Check sheet for the modelled part. Datum: model origin and axes. Units: mm. Round coordinates to 2 decimals unless told otherwise and drop trailing zeros. Loops run counter-clockwise (first coordinate to the right, second up) from the corner with the lowest first, then second, coordinate; pieces in that order, holes last. Notation, with made-up numbers: (67, -7) -> (106, -7) arc R21 ccw to (106, 29) -> close; hole circle Ø11 at (24, 15.5). An arc over 180 degrees is marked (long way). Return JSON: item names as keys, results as strings.
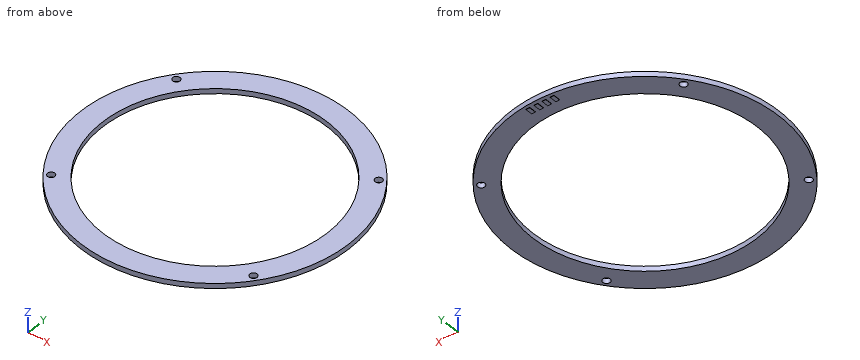
from build123d import *

# Parameters (mm, degrees)
SKETCH1_R           = 43
SKETCH1_R_2         = 36
SKETCH1_R_3         = 1.15
BOSS_EXTRUDE2_DEPTH = 1.6
SKETCH4_W           = 1.2
SKETCH4_H           = 2.3
BOSS_EXTRUDE3_DEPTH = 0.1


with BuildPart() as part:
    # Sketch1 → Boss-Extrude2 (new body)
    with BuildSketch(Plane.XY):
        Circle(SKETCH1_R)
        Circle(SKETCH1_R_2, mode=Mode.SUBTRACT)
        with Locations((32.5, -24.9)):
            Circle(SKETCH1_R_3, mode=Mode.SUBTRACT)
        with Locations((-32.5, -24.9)):
            Circle(SKETCH1_R_3, mode=Mode.SUBTRACT)
        with Locations((-32.5, 24.9)):
            Circle(SKETCH1_R_3, mode=Mode.SUBTRACT)
        with Locations((32.5, 24.9)):
            Circle(SKETCH1_R_3, mode=Mode.SUBTRACT)
    extrude(amount=BOSS_EXTRUDE2_DEPTH)

    # Sketch4 → Boss-Extrude3 (add)
    with BuildSketch(Plane(origin=(0, 0, 0), x_dir=(-1, 0, 0), z_dir=(0, 0, -1))):
        with Locations((1.3, 40.65)):
            Rectangle(SKETCH4_W, SKETCH4_H)
        with Locations((3.9, 40.65)):
            Rectangle(SKETCH4_W, SKETCH4_H)
        with Locations((-1.3, 40.65)):
            Rectangle(SKETCH4_W, SKETCH4_H)
        with Locations((-3.9, 40.65)):
            Rectangle(SKETCH4_W, SKETCH4_H)
    extrude(amount=BOSS_EXTRUDE3_DEPTH)


solid = part.part
Q1. Section check B-B (z = 0.65). Record the boundary of the cut face in (x, y), then the cut area to 3 significant figures.
Results list:
{"outline": "circle Ø86 at (0, 0); hole circle Ø72 at (0, 0); hole circle Ø2.3 at (-32.5, -24.9); hole circle Ø2.3 at (-32.5, 24.9); hole circle Ø2.3 at (32.5, -24.9); hole circle Ø2.3 at (32.5, 24.9)", "area": "1,720 mm^2"}
Q2. Section check D-D (y = 24.9). Record the boundary of the cut face in (x, z), then the cut area to 3 significant figures.
Results list:
{"outline": "(-35.06, 0) -> (-33.65, 0) -> (-33.65, 1.6) -> (-35.06, 1.6) -> close; (-31.35, 0) -> (-26, 0) -> (-26, 1.6) -> (-31.35, 1.6) -> close; (26, 0) -> (31.35, 0) -> (31.35, 1.6) -> (26, 1.6) -> close; (33.65, 0) -> (35.06, 0) -> (35.06, 1.6) -> (33.65, 1.6) -> close", "area": "21.6 mm^2"}
Q3. Section check A-A (y = 0). Record the boundary of the cut face in (x, z).
Results list:
{"outline": "(-43, 0) -> (-36, 0) -> (-36, 1.6) -> (-43, 1.6) -> close; (36, 0) -> (43, 0) -> (43, 1.6) -> (36, 1.6) -> close"}
Q4. Material ranges on line 1 (Y direction, x = 0, z = 0.6); line 2 (Y direction, x = -32.5, z = 1.15); line 3 (Y direction, x = 32, z = 1.5), recorded low to high.
Results list:
{"line 1": "-43 to -36, 36 to 43", "line 2": "-28.16 to -26.05, -23.75 to -15.48, 15.48 to 23.75, 26.05 to 28.16", "line 3": "-28.72 to -25.94, -23.86 to -16.49, 16.49 to 23.86, 25.94 to 28.72"}
Q5. Section check C-C (x = -28). Record the boundary of the cut face in (y, z).
Results list:
{"outline": "(-32.63, 0) -> (-22.63, 0) -> (-22.63, 1.6) -> (-32.63, 1.6) -> close; (22.63, 0) -> (32.63, 0) -> (32.63, 1.6) -> (22.63, 1.6) -> close"}
Q6. Go/stop test with a flat-tipped pin: pin 1 (3.5 mm diameter, centred on x = 32.5, y = 24.9, fed in from -Z). Record where the tip stops, or that it passes through.
Results list:
{"pin 1": "z = 0"}
